Design review of the part built by this model. Coordinates are the model's own, in mm. Coordinates: 2 decimals unless noted, no trailing zeros. Order: outer loops, then holes, each group sorted by start corner. A loop starts at its lowest first (then second) coordinate and runs counter-clockwise, first axis right, second up. Notation, with made-up numbers: M -35,49 L -30,49 A22 ccw -30,73 Z; hole C -6.75,64 d4. An arc over 180 degrees is marked long. Use CSV: the item, a comma, the result in double quotes.
```python
from build123d import *

# Parameters (mm, degrees)
SKETCH1_R           = 27.5
SKETCH1_R_2         = 2.65
BOSS_EXTRUDE1_DEPTH = 4
SKETCH2_R           = 7.25
CUT_EXTRUDE1_DEPTH  = 40.096035605


with BuildPart() as part:
    # Sketch1 → Boss-Extrude1 (new body)
    with BuildSketch(Plane.XY):
        Circle(SKETCH1_R)
        with Locations((0, 22.5)):
            Circle(SKETCH1_R_2, mode=Mode.SUBTRACT)
        with Locations((19.485571585, 11.25)):
            Circle(SKETCH1_R_2, mode=Mode.SUBTRACT)
        with Locations((19.485571585, -11.25)):
            Circle(SKETCH1_R_2, mode=Mode.SUBTRACT)
        with Locations((0, -22.5)):
            Circle(SKETCH1_R_2, mode=Mode.SUBTRACT)
        with Locations((-19.485571585, -11.25)):
            Circle(SKETCH1_R_2, mode=Mode.SUBTRACT)
        with Locations((-19.485571585, 11.25)):
            Circle(SKETCH1_R_2, mode=Mode.SUBTRACT)
    extrude(amount=BOSS_EXTRUDE1_DEPTH)

    # Sketch2 → Cut-Extrude1 (cut, through all)
    with BuildSketch(Plane.XY.offset(4)):
        Circle(SKETCH2_R)
    extrude(amount=-CUT_EXTRUDE1_DEPTH, mode=Mode.SUBTRACT)


solid = part.part
```
(1) Clearance check with flat-ended pins moving along their axes: P1, Ø1, axis at y = 15, z = 2, coming from the +X side; P2, Ø5, axis at x = 0, y = 22.5, coming from the -Z side; P3, Ø2, axis at x = 19, z = 1, coming from the -Y side. State where each tip first meets the part, or that it passes through.
The answers:
P1,"stops at x = 23.37"
P2,"passes through"
P3,"stops at y = -20.79"
(2) Add section C-C on y = 0. State the section outline as (x, z) points, and give its area (3 significant figures).
The answers:
outline,"M -27.5,0 L -7.25,0 L -7.25,4 L -27.5,4 Z; M 7.25,0 L 27.5,0 L 27.5,4 L 7.25,4 Z"
area,"162 mm2"
(3) Wall thickness on probe 1 along Y at (x, z) = (0, 1.25); probe 2 along Y at (x, z) = (18, 2.7); probe 3 along Y at (x, z) = (1.5, 2): over which ranges is each line inside the solid? List them lowest first.
The answers:
probe 1,"y = -27.5 to -25.15, -19.85 to -7.25, 7.25 to 19.85, 25.15 to 27.5"
probe 2,"y = -20.79 to -13.44, -9.06 to 9.06, 13.44 to 20.79"
probe 3,"y = -27.46 to -24.68, -20.32 to -7.09, 7.09 to 20.32, 24.68 to 27.46"
(4) Add section D-D on y = 12. State the section outline as (x, z) points, and give its area (3 significant figures).
The answers:
outline,"M -24.74,0 L -22.03,0 L -22.03,4 L -24.74,4 Z; M -16.94,0 L 16.94,0 L 16.94,4 L -16.94,4 Z; M 22.03,0 L 24.74,0 L 24.74,4 L 22.03,4 Z"
area,"157 mm2"
(5) Add section B-B on x = 0. State the section outline as (y, z) points.
The answers:
outline,"M -27.5,0 L -25.15,0 L -25.15,4 L -27.5,4 Z; M -19.85,0 L -7.25,0 L -7.25,4 L -19.85,4 Z; M 7.25,0 L 19.85,0 L 19.85,4 L 7.25,4 Z; M 25.15,0 L 27.5,0 L 27.5,4 L 25.15,4 Z"
(6) Add section A-A on z = 2.95. State the section outline as (x, y) points.
The answers:
outline,"C 0,0 d55; hole C -19.49,-11.25 d5.3; hole C -19.49,11.25 d5.3; hole C 0,0 d14.5; hole C 0,-22.5 d5.3; hole C 0,22.5 d5.3; hole C 19.49,-11.25 d5.3; hole C 19.49,11.25 d5.3"
(7) The part is to be moulded in two halves that separate along X. For faces 1 (the face through (21.933, 10.235, 1.972)), 2 (the face through (-5.961, -26.846, 1.972)), 3 (the face through (6, -6, 0)), say which applies: pulls with the +X half, pulls with the -X half, needs draft (parallel to the pull), parting line crosses it, or undercut.
The answers:
face 1,"undercut"
face 2,"parting line crosses it"
face 3,"needs draft"
